```python
from build123d import *

# Parameters (mm, degrees)
SKETCH2_W           = 10
SKETCH2_H           = 3.175
BOSS_EXTRUDE1_DEPTH = 3.175


with BuildPart() as part:
    # Sketch2 → Boss-Extrude1 (new body)
    with BuildSketch(Plane(origin=(0, 0, 0), x_dir=(1, 0, 0), z_dir=(0, 1, 0))):
        Polygon((-137.685687371, 51.939525879), (-137.685687371, 66.939525879), (114.314312629, 66.939525879), (114.314312629, 51.939525879), (117.489312629, 51.939525879), (117.489312629, 41.939525879), (114.314312629, 41.939525879), (114.314312629, 31.939525879), (117.489312629, 31.939525879), (117.489312629, 21.939525879), (114.314312629, 21.939525879), (114.314312629, 11.939525879), (117.489312629, 11.939525879), (117.489312629, 1.939525879), (114.314312629, 1.939525879), (114.314312629, -8.060474121), (117.489312629, -8.060474121), (117.489312629, -18.060474121), (114.314312629, -18.060474121), (114.314312629, -28.060474121), (117.489312629, -28.060474121), (117.489312629, -38.060474121), (114.314312629, -38.060474121), (114.314312629, -48.060474121), (117.489312629, -48.060474121), (117.489312629, -58.060474121), (114.314312629, -58.060474121), (114.314312629, -68.060474121), (117.489312629, -68.060474121), (117.489312629, -78.060474121), (114.314312629, -78.060474121), (114.314312629, -93.060474121), (-137.685687371, -93.060474121), (-137.685687371, -78.060474121), (-140.860687371, -78.060474121), (-140.860687371, -68.060474121), (-137.685687371, -68.060474121), (-137.685687371, -58.060474121), (-140.860687371, -58.060474121), (-140.860687371, -48.060474121), (-137.685687371, -48.060474121), (-137.685687371, -38.060474121), (-140.860687371, -38.060474121), (-140.860687371, -28.060474121), (-137.685687371, -28.060474121), (-137.685687371, -18.060474121), (-140.860687371, -18.060474121), (-140.860687371, -8.060474121), (-137.685687371, -8.060474121), (-137.685687371, 1.939525879), (-140.860687371, 1.939525879), (-140.860687371, 11.939525879), (-137.685687371, 11.939525879), (-137.685687371, 21.939525879), (-140.860687371, 21.939525879), (-140.860687371, 31.939525879), (-137.685687371, 31.939525879), (-137.685687371, 41.939525879), (-140.860687371, 41.939525879), (-140.860687371, 51.939525879), align=None)
        with Locations((-101.685687371, 62.352025879)):
            Rectangle(SKETCH2_W, SKETCH2_H, mode=Mode.SUBTRACT)
        with Locations((-121.685687371, 62.352025879)):
            Rectangle(SKETCH2_W, SKETCH2_H, mode=Mode.SUBTRACT)
        with Locations((-81.685687371, 62.352025879)):
            Rectangle(SKETCH2_W, SKETCH2_H, mode=Mode.SUBTRACT)
        with Locations((-61.685687371, 62.352025879)):
            Rectangle(SKETCH2_W, SKETCH2_H, mode=Mode.SUBTRACT)
        with Locations((-41.685687371, 62.352025879)):
            Rectangle(SKETCH2_W, SKETCH2_H, mode=Mode.SUBTRACT)
        with Locations((-21.685687371, 62.352025879)):
            Rectangle(SKETCH2_W, SKETCH2_H, mode=Mode.SUBTRACT)
        with Locations((-1.685687371, 62.352025879)):
            Rectangle(SKETCH2_W, SKETCH2_H, mode=Mode.SUBTRACT)
        with Locations((18.314312629, 62.352025879)):
            Rectangle(SKETCH2_W, SKETCH2_H, mode=Mode.SUBTRACT)
        with Locations((38.314312629, 62.352025879)):
            Rectangle(SKETCH2_W, SKETCH2_H, mode=Mode.SUBTRACT)
        with Locations((58.314312629, 62.352025879)):
            Rectangle(SKETCH2_W, SKETCH2_H, mode=Mode.SUBTRACT)
        with Locations((78.314312629, 62.352025879)):
            Rectangle(SKETCH2_W, SKETCH2_H, mode=Mode.SUBTRACT)
        with Locations((98.314312629, 62.352025879)):
            Rectangle(SKETCH2_W, SKETCH2_H, mode=Mode.SUBTRACT)
        with Locations((98.314312629, -88.472974121)):
            Rectangle(SKETCH2_W, SKETCH2_H, mode=Mode.SUBTRACT)
        with Locations((78.314312629, -88.472974121)):
            Rectangle(SKETCH2_W, SKETCH2_H, mode=Mode.SUBTRACT)
        with Locations((58.314312629, -88.472974121)):
            Rectangle(SKETCH2_W, SKETCH2_H, mode=Mode.SUBTRACT)
        with Locations((38.314312629, -88.472974121)):
            Rectangle(SKETCH2_W, SKETCH2_H, mode=Mode.SUBTRACT)
        with Locations((18.314312629, -88.472974121)):
            Rectangle(SKETCH2_W, SKETCH2_H, mode=Mode.SUBTRACT)
        with Locations((-1.685687371, -88.472974121)):
            Rectangle(SKETCH2_W, SKETCH2_H, mode=Mode.SUBTRACT)
        with Locations((-21.685687371, -88.472974121)):
            Rectangle(SKETCH2_W, SKETCH2_H, mode=Mode.SUBTRACT)
        with Locations((-41.685687371, -88.472974121)):
            Rectangle(SKETCH2_W, SKETCH2_H, mode=Mode.SUBTRACT)
        with Locations((-61.685687371, -88.472974121)):
            Rectangle(SKETCH2_W, SKETCH2_H, mode=Mode.SUBTRACT)
        with Locations((-81.685687371, -88.472974121)):
            Rectangle(SKETCH2_W, SKETCH2_H, mode=Mode.SUBTRACT)
        with Locations((-101.685687371, -88.472974121)):
            Rectangle(SKETCH2_W, SKETCH2_H, mode=Mode.SUBTRACT)
        with Locations((-121.685687371, -88.472974121)):
            Rectangle(SKETCH2_W, SKETCH2_H, mode=Mode.SUBTRACT)
    extrude(amount=BOSS_EXTRUDE1_DEPTH)


solid = part.part
```
Build history of the part. All positions in model axes, mm. Round coordinates to 2 decimals unless told otherwise and drop trailing zeros. Loops run counter-clockwise (first coordinate to the right, second up) from the corner with the lowest first, then second, coordinate; pieces in that order, holes last.
Item 1: Saw through at B-B (y = 1.4). State how many separate pieces and enclosed holes the cut face has, then the cut area to 3 significant figures.
Item 2: Pin check, flat tips, straight feed: P1, Ø1, axis at y = 1, z = -62, coming from the -X side; P2, Ø1, axis at y = 3, z = 6, coming from the +X side. Stop position of each tip, or through.
Item 3: Saw through at A-A (x = -82). List the corners of the cut face in (y, z) (3 decimals), then the cut area to 3 significant figures.
Item 4: Drill centre lines: line 1 along Z through (x, y) = (57, 2); line 2 along X through (y, z) = (2.4, 24). Where is each one in solid material? Low to high.
Worked answers:
1. separate pieces: 1
1. enclosed holes: 24
1. area: 40,000 mm2
2. P1: stops at x = -137.69
2. P2: stops at x = 114.31
3. outline: (0, -66.94) - (3.175, -66.94) - (3.175, -63.94) - (0, -63.94) - close; (0, -60.765) - (3.175, -60.765) - (3.175, 86.885) - (0, 86.885) - close; (0, 90.06) - (3.175, 90.06) - (3.175, 93.06) - (0, 93.06) - close
3. area: 488 mm2
4. line 1: z = -66.94 to -63.94, -60.76 to 86.89, 90.06 to 93.06
4. line 2: x = -137.69 to 114.31
